The listing builds one solid part. Answer for the finished solid, in the listing's coordinates (mm). Round coordinates to 2 decimals unless told otherwise and drop trailing zeros. Loops run counter-clockwise (first coordinate to the right, second up) from the corner with the lowest first, then second, coordinate; pieces in that order, holes last. Notation, with made-up numbers: (23, -5) - (80, -5) arc R19 ccw to (80, 8) - close; hole circle Ø11 at (27, 62.25). An arc over 180 degrees is marked (long way). One line per item, written item: value.
```python
from build123d import *

# Parameters (mm, degrees)
SKETCH_1_W      = 164
SKETCH_1_H      = 164
SKETCH_1_R      = 1.5
SKETCH_1_R_2    = 4.5
SKETCH_1_R_3    = 2
SKETCH_1_W_2    = 8.12
SKETCH_1_H_2    = 4.129008776
SKETCH_1_W_3    = 4.129008777
SKETCH_1_H_3    = 8.12
EXTRUDE_1_DEPTH = 4


with BuildPart() as part:
    # 草图1 → 凸台-拉伸1 (new body)
    with BuildSketch(Plane.XY):
        with Locations((47.027428163, 15.054738201)):
            Rectangle(SKETCH_1_W, SKETCH_1_H)
        with Locations((47.027428163, 90.054738201)):
            Circle(SKETCH_1_R, mode=Mode.SUBTRACT)
        with Locations((47.027428163, 15.054738201)):
            Circle(SKETCH_1_R_2, mode=Mode.SUBTRACT)
        with Locations((77.027428163, 90.054738201)):
            Circle(SKETCH_1_R, mode=Mode.SUBTRACT)
        with Locations((107.027428163, 90.054738201)):
            Circle(SKETCH_1_R, mode=Mode.SUBTRACT)
        with Locations((-12.972571837, 90.054738201)):
            Circle(SKETCH_1_R, mode=Mode.SUBTRACT)
        with Locations((67.027428163, 15.054738201)):
            Circle(SKETCH_1_R_3, mode=Mode.SUBTRACT)
        with Locations((17.027428163, 90.054738201)):
            Circle(SKETCH_1_R, mode=Mode.SUBTRACT)
        with Locations((122.027428163, 15.054738201)):
            Circle(SKETCH_1_R, mode=Mode.SUBTRACT)
        with Locations((122.027428163, -14.945261799)):
            Circle(SKETCH_1_R, mode=Mode.SUBTRACT)
        with Locations((122.027428163, -44.945261799)):
            Circle(SKETCH_1_R, mode=Mode.SUBTRACT)
        with Locations((122.027428163, 75.054738201)):
            Circle(SKETCH_1_R, mode=Mode.SUBTRACT)
        with Locations((67.027428163, 55.054738201)):
            Circle(SKETCH_1_R_3, mode=Mode.SUBTRACT)
        with Locations((122.027428163, 45.054738201)):
            Circle(SKETCH_1_R, mode=Mode.SUBTRACT)
        with Locations((47.027428163, -59.945261799)):
            Circle(SKETCH_1_R, mode=Mode.SUBTRACT)
        with Locations((17.027428163, -59.945261799)):
            Circle(SKETCH_1_R, mode=Mode.SUBTRACT)
        with Locations((-12.972571837, -59.945261799)):
            Circle(SKETCH_1_R, mode=Mode.SUBTRACT)
        with Locations((107.027428163, -59.945261799)):
            Circle(SKETCH_1_R, mode=Mode.SUBTRACT)
        with Locations((77.027428163, -59.945261799)):
            Circle(SKETCH_1_R, mode=Mode.SUBTRACT)
        with Locations((-27.972571837, 15.054738201)):
            Circle(SKETCH_1_R, mode=Mode.SUBTRACT)
        with Locations((-27.972571837, 45.054738201)):
            Circle(SKETCH_1_R, mode=Mode.SUBTRACT)
        with Locations((-27.972571837, 75.054738201)):
            Circle(SKETCH_1_R, mode=Mode.SUBTRACT)
        with Locations((-27.972571837, -44.945261799)):
            Circle(SKETCH_1_R, mode=Mode.SUBTRACT)
        with Locations((-27.972571837, -14.945261799)):
            Circle(SKETCH_1_R, mode=Mode.SUBTRACT)
        with Locations((27.027428163, 55.054738201)):
            Circle(SKETCH_1_R_3, mode=Mode.SUBTRACT)
        with Locations((27.027428163, 15.054738201)):
            Circle(SKETCH_1_R_3, mode=Mode.SUBTRACT)
        with Locations((47.027428163, 35.054738201)):
            Circle(SKETCH_1_R_3, mode=Mode.SUBTRACT)
        with Locations((62.027428163, 90.054738201)):
            Rectangle(SKETCH_1_W_2, SKETCH_1_H_2, mode=Mode.SUBTRACT)
        with Locations((92.027428163, 90.054738201)):
            Rectangle(SKETCH_1_W_2, SKETCH_1_H_2, mode=Mode.SUBTRACT)
        with Locations((2.027428163, 90.054738201)):
            Rectangle(SKETCH_1_W_2, SKETCH_1_H_2, mode=Mode.SUBTRACT)
        with Locations((32.027428163, 90.054738201)):
            Rectangle(SKETCH_1_W_2, SKETCH_1_H_2, mode=Mode.SUBTRACT)
        with Locations((122.027428164, 0.054738201)):
            Rectangle(SKETCH_1_W_3, SKETCH_1_H_3, mode=Mode.SUBTRACT)
        with Locations((122.027428164, -29.945261799)):
            Rectangle(SKETCH_1_W_3, SKETCH_1_H_3, mode=Mode.SUBTRACT)
        with Locations((122.027428164, 60.054738201)):
            Rectangle(SKETCH_1_W_3, SKETCH_1_H_3, mode=Mode.SUBTRACT)
        with Locations((122.027428164, 30.054738201)):
            Rectangle(SKETCH_1_W_3, SKETCH_1_H_3, mode=Mode.SUBTRACT)
        with Locations((32.027428163, -59.945261799)):
            Rectangle(SKETCH_1_W_2, SKETCH_1_H_2, mode=Mode.SUBTRACT)
        with Locations((2.027428163, -59.945261799)):
            Rectangle(SKETCH_1_W_2, SKETCH_1_H_2, mode=Mode.SUBTRACT)
        with Locations((92.027428163, -59.945261799)):
            Rectangle(SKETCH_1_W_2, SKETCH_1_H_2, mode=Mode.SUBTRACT)
        with Locations((62.027428163, -59.945261799)):
            Rectangle(SKETCH_1_W_2, SKETCH_1_H_2, mode=Mode.SUBTRACT)
        with Locations((-27.972571837, 30.054738201)):
            Rectangle(SKETCH_1_W_3, SKETCH_1_H_3, mode=Mode.SUBTRACT)
        with Locations((-27.972571837, 60.054738201)):
            Rectangle(SKETCH_1_W_3, SKETCH_1_H_3, mode=Mode.SUBTRACT)
        with Locations((-27.972571837, -29.945261799)):
            Rectangle(SKETCH_1_W_3, SKETCH_1_H_3, mode=Mode.SUBTRACT)
        with Locations((-27.972571837, 0.054738201)):
            Rectangle(SKETCH_1_W_3, SKETCH_1_H_3, mode=Mode.SUBTRACT)
    extrude(amount=EXTRUDE_1_DEPTH)


solid = part.part
```
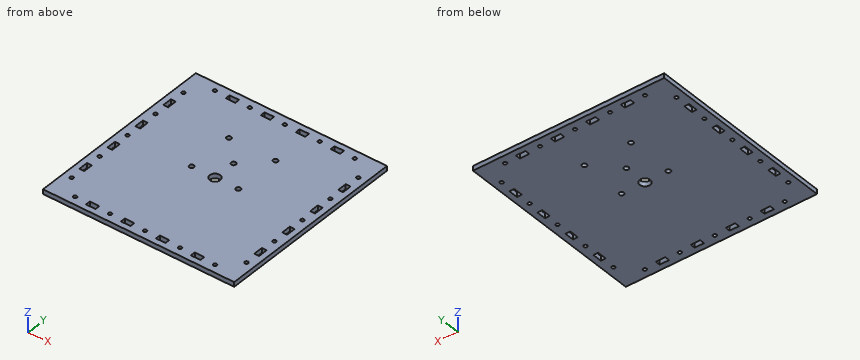
1) A cutting plane is placed at B-B on y = 60. Give the vertices of the cut face in (x, z), and give its area (3 significant figures).
Final values:
outline: (-34.97, 0) - (-30.04, 0) - (-30.04, 4) - (-34.97, 4) - close; (-25.91, 0) - (119.96, 0) - (119.96, 4) - (-25.91, 4) - close; (124.09, 0) - (129.03, 0) - (129.03, 4) - (124.09, 4) - close
area: 623 mm2
2) A cutting plane is placed at A-A on x = 31.5. Give the vertices of the cut face in (y, z), and give its area (3 significant figures).
Final values:
outline: (-66.95, 0) - (-62.01, 0) - (-62.01, 4) - (-66.95, 4) - close; (-57.88, 0) - (87.99, 0) - (87.99, 4) - (-57.88, 4) - close; (92.12, 0) - (97.05, 0) - (97.05, 4) - (92.12, 4) - close
area: 623 mm2
3) Each of these flat-tipped pins is pushed along its axis until it touches: pin 1 Ø6.5 at (x, y) = (27.03, 55.05) entering from -Z; pin 2 Ø2.5 at (x, y) = (-12.97, 90.05) entering from +Z. Where does it stop, or does it pass through?
Final values:
pin 1: z = 0
pin 2: through
4) Consider L1, parallel to Y at x = 0, z = 3.7; L2, parallel to X at y = 33.5, z = 2.5; L3, parallel to X at y = 46, z = 2.95. Determine where each line is inside the solid, lowest interval first.
Final values:
L1: -66.95 to -62.01, -57.88 to 87.99, 92.12 to 97.05
L2: -34.97 to -30.04, -25.91 to 45.77, 48.29 to 119.96, 124.09 to 129.03
L3: -34.97 to -29.14, -26.81 to 120.86, 123.19 to 129.03
5) A cutting plane is placed at C-C on z = 1.3. Give the number of separate pieces and of enclosed holes in the cut face, and give its area (3 significant figures).
Final values:
separate pieces: 1
enclosed holes: 42
area: 26,100 mm2
